The model under review builds one solid part; all positions refer to its coordinate system, in mm. Face numbers are marked on the shaded views. A direction names the side the tool comes from. Round coordinates to 2 decimals unless told otherwise and drop trailing zeros. Order: outer loops, then holes, each group sorted by start corner. A loop starts at its lowest first (then second) coordinate and runs counter-clockwise, first axis right, second up.
1) Machinability: for the marked faces 1, 2 and 3, which of the approach directions +Z, -Z, +X, -X, +Y, -Y give a long, thin tool a straight path to every point of the face, cutting with its end or side? Answer none if there is none.
2) Clearance check with flat-ended pins moving along their axes: P1, Ø8.5, axis at x = 20, z = -1, coming from the +Y side; P2, Ø5.5, axis at x = 0, z = 0.5, coming from the +Y side; P3, Ø1, axis at x = -17.5, y = 1, coming from the +Z side; P4, Ø2, axis at x = 14, y = 1, coming from the -Z side. State where each tip first meets the part, or that it passes through.
3) Consider section A-A (x = 0). Give the boundary of the cut face in (y, z).
4) To check wall thickness, follow L1, parallel to X at y = 0.6, z = 0; L2, parallel to Z at x = 17.5, y = 3.8; L3, parallel to X at y = 0.75, z = -0.75. State the ranges of each line that lie inside material, in increasing order.
5) Consider section B-B (z = 0). Give the number of separate pieces and of enclosed holes in the cut face, then the cut area to 3 significant figures.
6) Consider section D-D (y = 1.2). Give the boundary of the cut face in (x, z).
7) Consider section C-C (y = 3.1). Give the boundary of the cut face in (x, z), then the cut area to 3 significant figures.
8) Mouldability with a two-part tool opening along X and no side actions: class the marked faces 4 and 5 as pulls with the +X half, pulls with the -X half, needs draft (parallel to the pull), parting line crosses it, or undercut.
from build123d import *

# Parameters (mm, degrees)
SKETCH1_R           = 1.75
SKETCH1_R_2         = 4
BOSS_EXTRUDE1_DEPTH = 2
FILLET1_R           = 3
SKETCH2_R           = 5
SKETCH2_R_2         = 3
BOSS_EXTRUDE2_DEPTH = 3


with BuildPart() as part:
    # Sketch1 → Boss-Extrude1 (new body)
    # profile 1 of 5: a face of its own
    with BuildSketch(Plane(origin=(0, 0, 0), x_dir=(1, 0, 0), z_dir=(0, 1, 0))):
        with BuildLine():
            Line((-7.483314774, 5), (-25, 5))
            Line((-25, 5), (-25, -5))
            Line((-25, -5), (-7.483314774, -5))
            ThreePointArc((-7.483314774, -5), (-9, 0), (-7.483314774, 5))
        make_face()
        with Locations(Location((-17.5, 0, 0), (0, 0, 270))):
            Circle(SKETCH1_R, mode=Mode.SUBTRACT)
    # profile 2 of 5: a face of its own
    with BuildSketch(Plane(origin=(0, 0, 0), x_dir=(1, 0, 0), z_dir=(0, 1, 0))):
        with BuildLine():
            Line((7.483314774, -5), (-7.483314774, -5))
            ThreePointArc((-7.483314774, -5), (0, -9), (7.483314774, -5))
        make_face()
    # profile 3 of 5: a face of its own
    with BuildSketch(Plane(origin=(0, 0, 0), x_dir=(1, 0, 0), z_dir=(0, 1, 0))):
        with BuildLine():
            Line((7.483314774, 5), (-7.483314774, 5))
            ThreePointArc((-7.483314774, 5), (-9, 0), (-7.483314774, -5))
            Line((-7.483314774, -5), (7.483314774, -5))
            ThreePointArc((7.483314774, -5), (8.61248608, -2.61248608), (9, 0))
            ThreePointArc((9, 0), (8.61248608, 2.61248608), (7.483314774, 5))
        make_face()
        with Locations(Location((0, 0, 0), (0, 0, 270))):
            Circle(SKETCH1_R_2, mode=Mode.SUBTRACT)
    # profile 4 of 5: a face of its own
    with BuildSketch(Plane(origin=(0, 0, 0), x_dir=(1, 0, 0), z_dir=(0, 1, 0))):
        with BuildLine():
            ThreePointArc((7.483314774, 5), (0, 9), (-7.483314774, 5))
            Line((-7.483314774, 5), (7.483314774, 5))
        make_face()
    # profile 5 of 5: a face of its own
    with BuildSketch(Plane(origin=(0, 0, 0), x_dir=(1, 0, 0), z_dir=(0, 1, 0))):
        with BuildLine():
            Line((25, 5), (7.483314774, 5))
            ThreePointArc((7.483314774, 5), (8.61248608, 2.61248608), (9, 0))
            ThreePointArc((9, 0), (8.61248608, -2.61248608), (7.483314774, -5))
            Line((7.483314774, -5), (25, -5))
            Line((25, -5), (25, 5))
        make_face()
        with Locations(Location((17.5, 0, 0), (0, 0, 270))):
            Circle(SKETCH1_R, mode=Mode.SUBTRACT)
    extrude(amount=BOSS_EXTRUDE1_DEPTH)

    # Fillet1
    fillet1_edges = [part.edges().sort_by_distance(p)[0] for p in [
        (-25, 1, 5),
        (-25, 1, -5),
        (25, 1, -5),
        (25, 1, 5),
    ]]
    fillet(fillet1_edges, radius=FILLET1_R)

    # Sketch2 → Boss-Extrude2 (add)
    # profile 1 of 2: a face of its own
    with BuildSketch(Plane(origin=(0, 2, 0), x_dir=(1, 0, 0), z_dir=(0, 1, 0))):
        with Locations(Location((-17.5, 0, 0), (0, 0, 270))):
            Circle(SKETCH2_R)
        with Locations(Location((-17.5, 0, 0), (0, 0, 270))):
            Circle(SKETCH2_R_2, mode=Mode.SUBTRACT)
    # profile 2 of 2: a face of its own
    with BuildSketch(Plane(origin=(0, 2, 0), x_dir=(1, 0, 0), z_dir=(0, 1, 0))):
        with Locations(Location((17.5, 0, 0), (0, 0, 90))):
            Circle(SKETCH2_R)
        with Locations(Location((17.5, 0, 0), (0, 0, 90))):
            Circle(SKETCH2_R_2, mode=Mode.SUBTRACT)
    extrude(amount=BOSS_EXTRUDE2_DEPTH)


solid = part.part
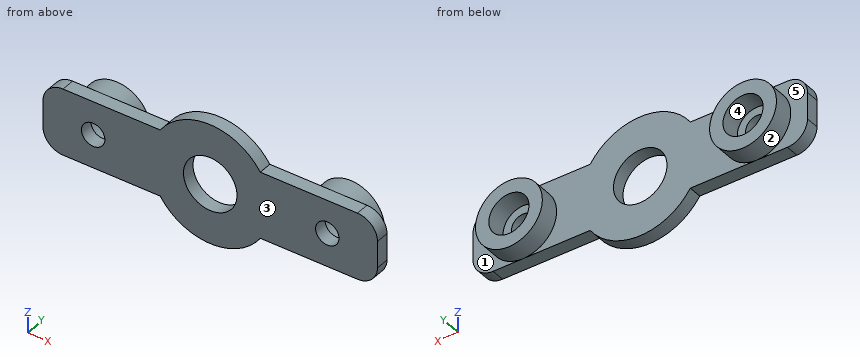
Answer below:
1. face 1: +X, +Y
1. face 2: +Y
1. face 3: +Z, -Z, +X, -X, -Y
2. P1: stops at y = 5
2. P2: passes through
2. P3: stops at z = 5
2. P4: stops at z = -5
3. outline: (0, -9) - (2, -9) - (2, -4) - (0, -4) - close; (0, 4) - (2, 4) - (2, 9) - (0, 9) - close
4. L1: x = -25 to -19.25, -15.75 to -4, 4 to 15.75, 19.25 to 25
4. L2: z = -5 to -3, 3 to 5
4. L3: x = -25 to -19.08, -15.92 to -3.93, 3.93 to 15.92, 19.08 to 25
5. separate pieces: 4
5. enclosed holes: 0
5. area: 94.0 mm2
6. outline: (-25, -2) arc R3 ccw to (-22, -5) - (-7.48, -5) arc R9 ccw to (7.48, -5) - (22, -5) arc R3 ccw to (25, -2) - (25, 2) arc R3 ccw to (22, 5) - (7.48, 5) arc R9 ccw to (-7.48, 5) - (-22, 5) arc R3 ccw to (-25, 2) - close; hole circle Ø3.5 at (-17.5, 0); hole circle Ø8 at (0, 0); hole circle Ø3.5 at (17.5, 0)
7. outline: circle Ø10 at (-17.5, 0); circle Ø10 at (17.5, 0); hole circle Ø6 at (-17.5, 0); hole circle Ø6 at (17.5, 0)
7. area: 101 mm2
8. face 4: undercut
8. face 5: needs draft
